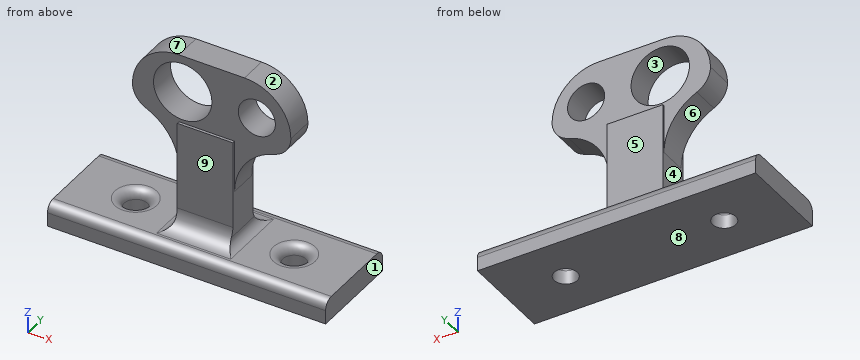
```python
from build123d import *

# Parameters (mm, degrees)
ESBO_O1_W                     = 60
ESBO_O1_H                     = 20
ESBO_O1_R                     = 2.5
RESSALTO_EXTRUS_O2_DEPTH      = 5
ESBO_O2_W                     = 12
ESBO_O2_H                     = 7
RESSALTO_EXTRUS_O3_DEPTH      = 28
RESSALTO_EXTRUS_O4_DEPTH      = 3
RESSALTO_EXTRUS_O4_DEPTH_BACK = 3
ESBO_O3_R                     = 4
ESBO_O3_R_2                   = 6.3
FILETE1_R                     = 10
FILETE2_R                     = 10
FILETE5_R                     = 5
FILETE7_R                     = 5
FILETE9_R                     = 2
FILETE10_R                    = 2
FILETE13_R                    = 12
FILETE14_R                    = 12
FILETE15_R                    = 4
FILETE16_R                    = 4
FILETE17_R                    = 2
FILETE18_R                    = 2
FILETE19_R                    = 2
FILETE20_R                    = 2


with BuildPart() as part:
    # Esboço1 → Ressalto-extrusão2 (new body)
    with BuildSketch(Plane.XY):
        with Locations((3.626373626, -0.10989011)):
            Rectangle(ESBO_O1_W, ESBO_O1_H)
        with Locations((-13.473626374, -0.10989011)):
            Circle(ESBO_O1_R, mode=Mode.SUBTRACT)
        with Locations((20.726373626, -0.10989011)):
            Circle(ESBO_O1_R, mode=Mode.SUBTRACT)
    extrude(amount=RESSALTO_EXTRUS_O2_DEPTH)

    # Esboço2 → Ressalto-extrusão3 (add)
    with BuildSketch(Plane.XY):
        with Locations((3.626373626, -0.10989011)):
            Rectangle(ESBO_O2_W, ESBO_O2_H)
    extrude(amount=RESSALTO_EXTRUS_O3_DEPTH)

    # Esboço3 → Ressalto-extrusão4 (add, two sides: drawn at the far end of the back side and taken through both)
    with BuildSketch(Plane(origin=(0, 0, 0), x_dir=(1, 0, 0), z_dir=(0, 1, 0)).offset(-RESSALTO_EXTRUS_O4_DEPTH_BACK)):
        Polygon((-21.373626374, -43), (28.626373626, -43), (20.428395134, -28), (-11.066061454, -28), align=None)
        with Locations(Location((14.428395134, -35, 0), (0, 0, 270))):
            Circle(ESBO_O3_R, mode=Mode.SUBTRACT)
        with Locations(Location((-1.571604866, -35, 0), (0, 0, 270))):
            Circle(ESBO_O3_R_2, mode=Mode.SUBTRACT)
    extrude(amount=RESSALTO_EXTRUS_O4_DEPTH + RESSALTO_EXTRUS_O4_DEPTH_BACK)

    # Filete1
    # the kernel refuses this fillet: 10 mm, written as the material it takes off along each edge
    with BuildSketch(Plane(origin=(-21.373626374, 50.419547395, 43), x_dir=(0.5663446817088761, 0, -0.8241684909653315), z_dir=(0, -1, 0))) as filete1_piece_1:
        with BuildLine():
            CenterArc((18.9840083, 9.96923191), FILETE1_R, 145.504279398, 120)
            Line((10.74232339, 15.632678727), (10.577489692, 15.745947664))
            Line((10.577489692, 15.745947664), (-0.164833698, 0.113268936))
            Line((-0.164833698, 0.113268936), (0, -0.2))
            ThreePointArc((0, -0.2), (9.100080969, -0.2), (18.184485011, -0.199384638))
            Line((18.184485011, -0.199384638), (18.200161938, 0))
        make_face()
    extrude(amount=100.839094789, mode=Mode.SUBTRACT)

    # Filete2
    filete2_edges = [part.edges().sort_by_distance(p)[0] for p in [
        (28.626373626, 0, 43),
    ]]
    fillet(filete2_edges, radius=FILETE2_R)

    # Filete5
    filete5_edges = [part.edges().sort_by_distance(p)[0] for p in [
        (20.428395134, 0, 28),
    ]]
    fillet(filete5_edges, radius=FILETE5_R)

    # Filete7
    filete7_edges = [part.edges().sort_by_distance(p)[0] for p in [
        (-11.066061454, 0, 28),
    ]]
    fillet(filete7_edges, radius=FILETE7_R)

    # Filete9
    filete9_edges = [part.edges().sort_by_distance(p)[0] for p in [
        (9.626373626, -0.10989011, 5),
    ]]
    fillet(filete9_edges, radius=FILETE9_R)

    # Filete10
    filete10_edges = [part.edges().sort_by_distance(p)[0] for p in [
        (-2.373626374, -0.10989011, 5),
    ]]
    fillet(filete10_edges, radius=FILETE10_R)

    # Filete13
    # the kernel refuses this fillet: 12 mm, written as the material it adds along each edge
    with BuildSketch(Plane(origin=(-2.373626374, -3, 28), x_dir=(0, 0, -1), z_dir=(0, 1, 0))) as filete13_piece_1_section:
        with BuildLine():
            CenterArc((10.506434115, 12), FILETE13_R, 204.196775666, 65.803224334)
            Line((-0.439284084, 7.081539559), (-1.533855904, 6.589693515))
            ThreePointArc((-1.533855904, 6.589693515), (-1.2, 5.032181042), (-1.2, 0))
            Line((-1.2, 0), (0, -1.2))
            Line((0, -1.2), (10.506434115, -1.2))
            Line((10.506434115, -1.2), (10.506434115, 0))
        make_face()
    filete13_piece_1 = extrude(amount=6, mode=Mode.PRIVATE)
    filete13_piece_1 = filete13_piece_1 - Plane(origin=(-1.571604866, 0, 35), x_dir=(0, 0, 1), z_dir=(0, -1, 0)) * Cylinder(6.3, 55, mode=Mode.PRIVATE)
    add(filete13_piece_1)

    # Filete14
    # the kernel refuses this fillet: 12 mm, written as the material it adds along each edge
    with BuildSketch(Plane(origin=(9.626373626, 3, 28), x_dir=(0.9997032338035666, 0, 0.02436071268849559), z_dir=(0, -1, 0))) as filete14_piece_1:
        with BuildLine():
            CenterArc((11.721404045, -11.579073047), FILETE14_R, 105.220471519, 73.38362437)
            Line((-0.275034761, -11.286744494), (-1.474678641, -11.257511639))
            Line((-1.474678641, -11.257511639), (-1.199643881, 0.029232855))
            Line((-1.199643881, 0.029232855), (0.029232855, 1.199643881))
            ThreePointArc((0.029232855, 1.199643881), (7.165756053, 1.025741481), (8.255955801, 1.157907305))
            Line((8.255955801, 1.157907305), (8.570996551, 0))
        make_face()
    extrude(amount=6)

    # Filete15
    filete15_edges = [part.edges().sort_by_distance(p)[0] for p in [
        (3.626373626, 3.39010989, 5),
    ]]
    fillet(filete15_edges, radius=FILETE15_R)

    # Filete16
    filete16_edges = [part.edges().sort_by_distance(p)[0] for p in [
        (3.626373626, -3.60989011, 5),
    ]]
    fillet(filete16_edges, radius=FILETE16_R)

    # Filete17
    filete17_edges = [part.edges().sort_by_distance(p)[0] for p in [
        (18.226373626, -0.10989011, 5),
    ]]
    fillet(filete17_edges, radius=FILETE17_R)

    # Filete18
    filete18_edges = [part.edges().sort_by_distance(p)[0] for p in [
        (-15.973626374, -0.10989011, 5),
    ]]
    fillet(filete18_edges, radius=FILETE18_R)

    # Filete19
    filete19_edges = [part.edges().sort_by_distance(p)[0] for p in [
        (3.626373626, 9.89010989, 5),
    ]]
    fillet(filete19_edges, radius=FILETE19_R)

    # Filete20
    filete20_edges = [part.edges().sort_by_distance(p)[0] for p in [
        (3.626373626, -10.10989011, 5),
    ]]
    fillet(filete20_edges, radius=FILETE20_R)


solid = part.part
```
Build history of the part. All positions in model axes, mm. Face numbers are marked on the shaded views. A direction names the side the tool comes from. Give positions to 0.01 mm unless a question says otherwise; leave off trailing zeros. Order: outer loops, then holes, each group sorted by start corner. A loop starts at its lowest first (then second) coordinate and runs counter-clockwise, first axis right, second up. Notation, with made-up numbers: M 34.25,21 L 81.25,21 A28 ccw 81.25,40 Z; hole C 56,-1 d1. An arc over 180 degrees is marked long. Write item = value, one per line. Start each with the question number.
(1) Slice it at A-A on x = 1. Write the cut outline in (y, z).
(2) Slice it at D-D on z = 25. Write the cut outline in (x, y).
(3) Slice it at B-B on z = 38. Write the cut outline in (x, y).
(4) Two-plate mould, pull along Z, no slides. Class the marked faces 1, 2, 3 and 4: released by +Z, released by -Z, zero draft, split by the parting line, or undercut.
(5) Which spindle directions (+Z, -Z, +X, -X, +Y, -Y) get a long thin tool onto all of the face, cutting with end or side? Do the marked faces 5, 6, 7, 8 and 9. Say none if no direction does.
(6) Probe L1, parallel to Z at x = 14.5, y = 2; L2, parallel to X at y = -1.4, z = 35; L3, parallel to Y at x = 2.5, z = 16.5. List the from-to ranges inside material, lowest first. Write a range as [from, to].
(7) Slice it at C-C on x = -6.5. Write the cut outline in (y, z).
(8) Pin check, flat tips, straight feed: pin 1 Ø10 at (x, z) = (-10.5, 23) entering from -Y; pin 2 Ø13 at (x, z) = (5.5, 35.5) entering from -Y; pin 3 Ø1.5 at (x, z) = (11.5, 28.5) entering from +Y; pin 4 Ø6.5 at (y, z) = (1.5, 17.5) entering from +X. Stop position of each tip, or through.
Responses:
q1.outline = M -10.11,0 L 9.89,0 L 9.89,3 A2 ccw 7.89,5 L 7.39,5 A4 cw 3.39,9 L 3.39,28 L 3,28 L 3,29.25 L -3,29.25 L -3,28 L -3.61,28 L -3.61,9 A4 cw -7.61,5 L -8.11,5 A2 ccw -10.11,3 Z; M -3,40.75 L 3,40.75 L 3,43 L -3,43 Z
q2.outline = M -5.01,-3 L -2.37,-3 L -2.37,-3.61 L 9.63,-3.61 L 9.63,-3 L 12.95,-3 L 12.95,3 L 9.63,3 L 9.63,3.39 L -2.37,3.39 L -2.37,3 L -5.01,3 Z
q3.outline = M -11.07,-3 L -7.11,-3 L -7.11,3 L -11.07,3 Z; M 3.97,-3 L 11.78,-3 L 11.78,3 L 3.97,3 Z; M 17.07,-3 L 20.43,-3 L 20.43,3 L 17.07,3 Z
q4.face_1 = zero draft
q4.face_2 = released by +Z
q4.face_3 = undercut
q4.face_4 = undercut
q5.face_5 = +Z, +X, -X, +Y
q5.face_6 = -X, +Y, -Y
q5.face_7 = +Z, -X, +Y, -Y
q5.face_8 = -Z, +X, -X, +Y, -Y
q5.face_9 = +Z, +X, -X, -Y
q6.L1 = [0, 5], [26.36, 31], [39, 42.62]
q6.L2 = [-12.2, -7.87], [4.73, 10.43], [18.43, 21.56]
q6.L3 = [-3.61, 3.39]
q7.outline = M -10.11,0 L 9.89,0 L 9.89,3 A2 ccw 7.89,5 L -8.11,5 A2 ccw -10.11,3 Z; M -3,26.55 L 3,26.55 L 3,31.08 L -3,31.08 Z; M -3,38.92 L 3,38.92 L 3,42.12 L -3,42.12 Z
q8.pin_1 = through
q8.pin_2 = -3
q8.pin_3 = 3
q8.pin_4 = 10.33
